from build123d import *

# Parameters (mm, degrees)
F0_W     = 12.5
F0_H     = 5.4
F1_DEPTH = 18
F2_R     = 2
F3_DEPTH = 34.501
F4_W     = 5
F4_H     = 16.2
F5_DEPTH = 2
F6_W     = 5.4
F6_H     = 11
F7_DEPTH = 47.001
F9_DEPTH = 16.201


with BuildPart() as f1:
    # F0 (on Top) → F1 (new body)
    with BuildSketch(Plane.XY):
        Polygon((11, 0), (0, 0), (-11, 0), (-11, -5.4), (-11, -16.2), (0, -16.2), (11, -16.2), (11, -5.4), align=None)
        with Locations((17.25, -2.7)):
            Rectangle(F0_W, F0_H)
        with Locations((-17.25, -2.7)):
            Rectangle(F0_W, F0_H)
    extrude(amount=F1_DEPTH)

    # F2 (on face) → F3 (cut, through all)
    with BuildSketch(Plane.YZ.offset(11)):
        with Locations((-11.2, 2.3)):
            Circle(F2_R)
    extrude(amount=-F3_DEPTH, mode=Mode.SUBTRACT)

    # F4 (on face) → F5 (join)
    with BuildSketch(Plane(origin=(0, 0, 0), x_dir=(1, 0, 0), z_dir=(0, 0, -1))):
        with Locations((2.5, 8.1)):
            Rectangle(F4_W, F4_H)
        with Locations((-2.5, 8.1)):
            Rectangle(F4_W, F4_H)
    extrude(amount=F5_DEPTH)

    # F6 (on face) → F7 (cut, through all)
    with BuildSketch(Plane.YZ.offset(23.5)):
        with Locations((-2.7, 12.5)):
            Rectangle(F6_W, F6_H)
    extrude(amount=-F7_DEPTH, mode=Mode.SUBTRACT)

    # F8 (on face) → F9 (cut, through all)
    with BuildSketch(Plane.XZ.offset(16.2)):
        Polygon((2.5, 18), (0, 18), (-2.5, 18), (-2.5, 15.5), (2.5, 15.5), align=None)
    extrude(amount=-F9_DEPTH, mode=Mode.SUBTRACT)


solid = f1.part
CAD build for the part. Positions are in the model's coordinates, mm. A direction names the side the tool comes from. Coordinates: 2 decimals unless noted, no trailing zeros. Loops run counter-clockwise (first coordinate to the right, second up) from the corner with the lowest first, then second, coordinate; pieces in that order, holes last. Notation, with made-up numbers: (-27.75, -13) - (9.25, -13) arc R27 cw to (9.25, 11) - close; hole circle Ø6 at (-14.5, -7.75). An arc over 180 degrees is marked (long way). Use one line per item in the form item = value. Start each with the question number.
1) Band-saw the part on A-A (y = -11.2). Give the cut face in (x, z).
2) Band-saw the part on D-D (y = -4.25). Give the cut face in (x, z).
3) Drill centre lines: L1, parallel to Z at x = 0, y = -11.2; L2, parallel to Z at x = -3.25, y = -11.2; L3, parallel to X at y = -8.25, z = 7.75. Where is each one in solid material? Low to high. Write a range as from..to.
4) Tool access for faces 1 (the face through (5, -8, -1)), 2 (the face through (-12, -4, 0)), 3 (the face through (-11, -11, 9)), 4 (the face through (0, -3, 7)): list every direction of +Z, -Z, +X, -X, +Y, -Y with a clear straight run to the whole face (end or side of a thin tool).
5) Band-saw the part on C-C (x = -3). Give the cut face in (y, z).
6) Flat gauge pins, fed straight in: pin 1 (3.5 mm diameter, centred on x = 15, z = 3.5, fed in from -Y); pin 2 (0.8 mm diameter, centred on y = -12.5, z = 17, fed in from +X); pin 3 (3 mm diameter, centred on y = -10, z = 11.5, fed in from -X). Where does each tip first touch, or does it go through?
7) Band-saw the part on B-B (z = 2.3). Give the cut face in (x, y).
8) Two-plate mould, pull along X, no slides. Class faces 5 (the face through (7, -11, 18)), 6 (the face through (-2.5, -11, 17)), 7 (the face through (0, -11, 15.5)), 8 (the face through (-5, -8, -1)): +X half, -X half, draft (parallel to the pull), parting line (faces both ways), or undercut.
Check values:
q1.outline = (-11, 0) - (-5, 0) - (-5, -2) - (5, -2) - (5, 0) - (11, 0) - (11, 0.3) - (-11, 0.3) - close; (-11, 4.3) - (11, 4.3) - (11, 18) - (2.5, 18) - (2.5, 15.5) - (-2.5, 15.5) - (-2.5, 18) - (-11, 18) - close
q2.outline = (-23.5, 0) - (-5, 0) - (-5, -2) - (5, -2) - (5, 0) - (23.5, 0) - (23.5, 7) - (-23.5, 7) - close
q3.L1 = -2..0.3, 4.3..15.5
q3.L2 = -2..0.3, 4.3..18
q3.L3 = -11..11
q4.face_1 = -Z, +X, +Y, -Y
q4.face_2 = -Z, -X, +Y, -Y
q4.face_3 = +Z, -Z, -X, -Y
q4.face_4 = +Z, +X, -X, +Y
q5.outline = (-16.2, -2) - (0, -2) - (0, 7) - (-5.4, 7) - (-5.4, 18) - (-16.2, 18) - close; hole circle Ø4 at (-11.2, 2.3)
q6.pin_1 = -5.4
q6.pin_2 = 11
q6.pin_3 = -11
q7.outline = (-23.5, -5.4) - (-11, -5.4) - (-11, -9.2) - (11, -9.2) - (11, -5.4) - (23.5, -5.4) - (23.5, 0) - (-23.5, 0) - close; (-11, -16.2) - (11, -16.2) - (11, -13.2) - (-11, -13.2) - close
q8.face_5 = draft
q8.face_6 = undercut
q8.face_7 = undercut
q8.face_8 = -X half
